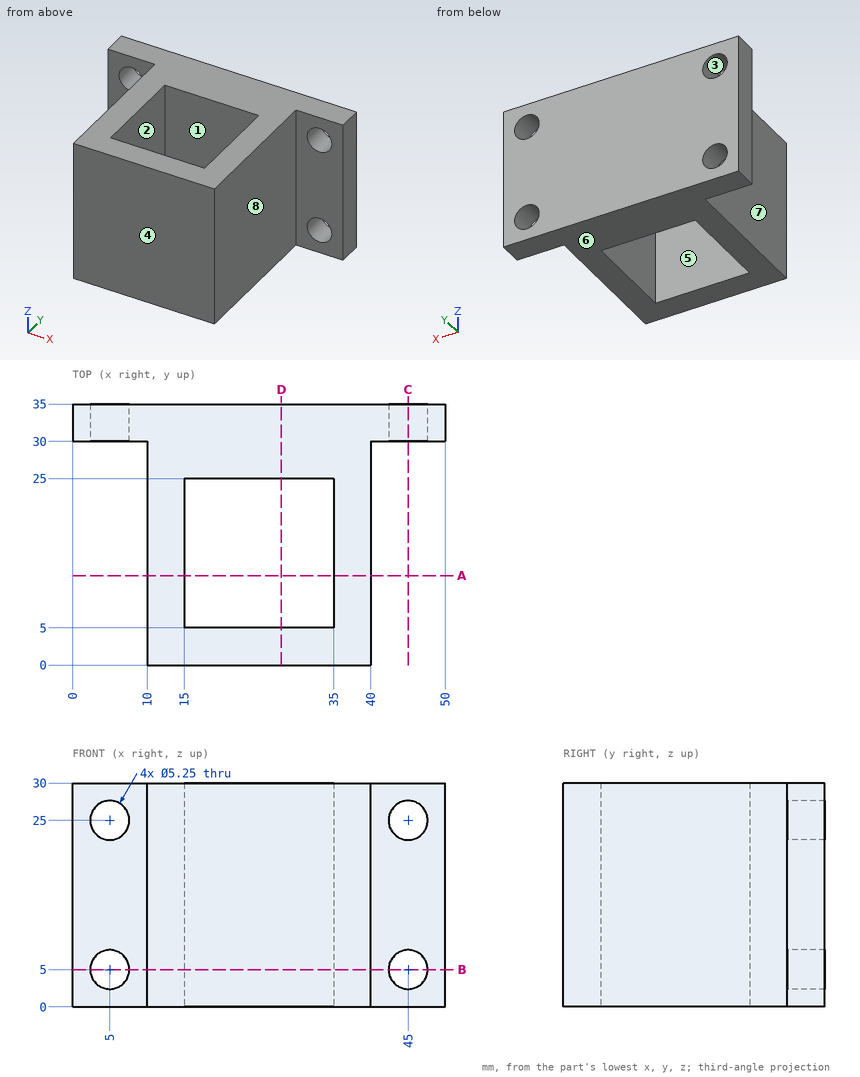
Could you check a few things on this drawing? It's one solid part, dimensions in mm from its lowest x, y, z. A direction names the side the tool comes from. Coordinates: 2 decimals unless noted, no trailing zeros. Order: outer loops, then holes, each group sorted by start corner. A loop starts at its lowest first (then second) coordinate and runs counter-clockwise, first axis right, second up.
1) I need wall thicknesses on line 1 (Z direction, x = 5, y = 33) (3 decimals); line 2 (X direction, y = 20, z = 22.5); line 3 (Y direction, x = 32.5, z = 20.25). Which ranges of each line are inside material? Lowest first, please.
2) Imagine slicing it at A-A on y = 12. List the corners of the cut face in (x, z) for me.
3) Imagine slicing it at D-D on x = 28. List the corners of the cut face in (y, z) for me.
4) Which directions (+Z, -Z, +X, -X, +Y, -Y) give clear straight access to the entire face, cutting with the end or side of a thin tool? Please do the marked faces 5, 6, 7 and 8.
5) We'd pull the mould along Y, two halves only. Please class the marked faces 1, 2, 3 and 4: +Y half, -Y half, draft (parallel to the pull), parting line (faces both ways), or undercut.
6) Imagine slicing it at C-C on x = 45. List the corners of the cut face in (y, z) for me (3 decimals), and give its area (3 significant figures).
7) Imagine slicing it at B-B on z = 5. List the corners of the cut face in (x, y) for me (3 decimals), and give its area (4 significant figures).
8) Will these pins go through, and if not, where does the flat tip stop? pin 1 (8 mm diameter, centred on y = 20, z = 25.5, fed in from +X); pin 2 (5 mm diameter, centred on x = 42, z = 18.5, fed in from -Y); pin 3 (4.5 mm diameter, centred on x = 5, z = 25, fed in from +Y) (3 decimals); pin 4 (6 mm diameter, centred on x = 45, z = 5, fed in from -Y).
Response values:
1. line 1: z = 0 to 2.375, 7.625 to 22.375, 27.625 to 30
1. line 2: x = 10 to 15, 35 to 40
1. line 3: y = 0 to 5, 25 to 35
2. outline: (10, 0) - (15, 0) - (15, 30) - (10, 30) - close; (35, 0) - (40, 0) - (40, 30) - (35, 30) - close
3. outline: (0, 0) - (5, 0) - (5, 30) - (0, 30) - close; (25, 0) - (35, 0) - (35, 30) - (25, 30) - close
4. face 5: +Z, -Z
4. face 6: -Z, +X, -X, +Y, -Y
4. face 7: +Z, -Z, -X, -Y
4. face 8: +Z, -Z, +X, -Y
5. face 1: undercut
5. face 2: undercut
5. face 3: draft
5. face 4: -Y half
6. outline: (30, 0) - (35, 0) - (35, 2.375) - (30, 2.375) - close; (30, 7.625) - (35, 7.625) - (35, 22.375) - (30, 22.375) - close; (30, 27.625) - (35, 27.625) - (35, 30) - (30, 30) - close
6. area: 97.5 mm2
7. outline: (0, 30) - (2.375, 30) - (2.375, 35) - (0, 35) - close; (7.625, 30) - (10, 30) - (10, 0) - (40, 0) - (40, 30) - (42.375, 30) - (42.375, 35) - (7.625, 35) - close; (47.625, 30) - (50, 30) - (50, 35) - (47.625, 35) - close; hole (15, 5) - (35, 5) - (35, 25) - (15, 25) - close
7. area: 697.5 mm2
8. pin 1: stops at x = 40
8. pin 2: stops at y = 0
8. pin 3: passes through
8. pin 4: stops at y = 30
